```python
from build123d import *

# Parameters (mm, degrees)
F1_DEPTH = 12.7
F3_DEPTH = 12.7
F5_DEPTH = 12.7


with BuildPart() as f1:
    # F0 (on Right) → F1 (new body)
    with BuildSketch(Plane.YZ):
        Polygon((-12.7, 12.7), (-12.7, 0), (12.7, 0), (12.7, 25.4), (0, 25.4), align=None)
    extrude(amount=-F1_DEPTH)

    # F2 (on face) → F3 (join)
    with BuildSketch(Plane(origin=(0, 0, 0), x_dir=(1, 0, 0), z_dir=(0, 0, -1))):
        Polygon((-38.1, -12.7), (-12.7, -12.7), (-12.7, -6.35), (-25.4, -6.35), (-25.4, 0), (-38.1, 0), align=None)
    extrude(amount=-F3_DEPTH)

    # F4 (on face) → F5 (join)
    with BuildSketch(Plane(origin=(-38.1, 0, 0), x_dir=(0, -1, 0), z_dir=(-1, 0, 0))):
        Polygon((12.7, 0), (0, 12.7), (0, 0), align=None)
    extrude(amount=-F5_DEPTH)


solid = f1.part
```
Verification items for the finished model (mm, model axes). A direction names the side the tool comes from. Give positions to 0.01 mm unless a question says otherwise; leave off trailing zeros. Order: outer loops, then holes, each group sorted by start corner. A loop starts at its lowest first (then second) coordinate and runs counter-clockwise, first axis right, second up. Notation, with made-up numbers: (73.25, 39.25) -> (127.25, 39.25) arc R9 ccw to (127.25, 48.25) -> close; hole circle Ø10 at (-0.75, 48). An arc over 180 degrees is marked (long way). Use a Markdown table: item, result.
1) Tool access check on faces 4 (the flat face through (-19, 6.35, 6)), 5 (the flat face through (-31.8, -6.4, 6.3)), 6 (the flat face through (-28, 8, 12.7)), 7 (the flat face through (-12.7, 0, 13)). Record the directions out of +Z, -Z, +X, -X, +Y, -Y that give a thin tool (end or side, any length) a straight path to the whole face; none if there is none.
Results:
| item | result |
|---|---|
| face 4 | +Z, -Z, -Y |
| face 5 | +Z, -X, -Y |
| face 6 | +Z, -X, +Y, -Y |
| face 7 | +Z, -Y |
2) Section check C-C, the plane x = -12. Record the boundary of the cut face in (y, z).
Results:
| item | result |
|---|---|
| outline | (-12.7, 0) -> (12.7, 0) -> (12.7, 25.4) -> (0, 25.4) -> (-12.7, 12.7) -> close |
3) Mould release check, pull along X, two halves, no side actions. Record for faces 1 (the flat face through (0, 0, 13)), 2 (the flat face through (-6, -12.7, 6)), 3 (the flat face through (-25.4, -1, 5)): pulls with the +X half, pulls with the -X half, needs draft (parallel to the pull), parting line crosses it, or undercut.
Results:
| item | result |
|---|---|
| face 1 | pulls with the +X half |
| face 2 | needs draft |
| face 3 | undercut |
4) Section check A-A, the plane y = -5.5. Record the boundary of the cut face in (x, z), then the cut area to 3 significant figures.
Results:
| item | result |
|---|---|
| outline | (-38.1, 0) -> (-25.4, 0) -> (-25.4, 7.2) -> (-38.1, 7.2) -> close; (-12.7, 0) -> (0, 0) -> (0, 19.9) -> (-12.7, 19.9) -> close |
| area | 344 mm² |
5) Depth check by flat-ended pin: pin 1 Ø4 at (x, y) = (-19.5, 8.5) entering from +Z; pin 2 Ø6.5 at (x, z) = (-21, 4.5) entering from -Y; pin 3 Ø5 at (x, y) = (-5.5, -6) entering from +Z; pin 4 Ø5 at (x, y) = (-21, -8) entering from +Z. Enter the tip coordinate at first touch or a pass-through.
Results:
| item | result |
|---|---|
| pin 1 | z = 12.7 |
| pin 2 | y = 6.35 |
| pin 3 | z = 21.9 |
| pin 4 | through |
6) Material ranges on probe 1 along X at (y, z) = (-2, 2.5); probe 2 along X at (y, z) = (10, 15.5); probe 3 along Z at (x, y) = (-14, 10.5), recorded low to high.
Results:
| item | result |
|---|---|
| probe 1 | -38.1 to -25.4, -12.7 to 0 |
| probe 2 | -12.7 to 0 |
| probe 3 | 0 to 12.7 |
7) Section check D-D, the plane y = 2.75. Record the boundary of the cut face in (x, z), then the cut area to 3 significant figures.
Results:
| item | result |
|---|---|
| outline | (-38.1, 0) -> (-25.4, 0) -> (-25.4, 12.7) -> (-38.1, 12.7) -> close; (-12.7, 0) -> (0, 0) -> (0, 25.4) -> (-12.7, 25.4) -> close |
| area | 484 mm² |
8) Section check B-B, the plane z = 9.5. Record the boundary of the cut face in (x, y), then the cut area to 3 significant figures.
Results:
| item | result |
|---|---|
| outline | (-38.1, -3.2) -> (-25.4, -3.2) -> (-25.4, 6.35) -> (-12.7, 6.35) -> (-12.7, -12.7) -> (0, -12.7) -> (0, 12.7) -> (-38.1, 12.7) -> close |
| area | 605 mm² |
